Model file for the job. Use its own axes, mm. A direction names the side the tool comes from. Give positions to 0.01 mm unless a question says otherwise; leave off trailing zeros. Order: outer loops, then holes, each group sorted by start corner. A loop starts at its lowest first (then second) coordinate and runs counter-clockwise, first axis right, second up. Notation, with made-up numbers: M 64,22.25 L 116,22.25 A4 ccw 116,29.25 Z; hole C -8.5,48.25 d10. An arc over 180 degrees is marked long. Return JSON: item names as keys, results as strings. Group by question number.
1. Slice it at A-A on z = 4. List the corners of the cut face in (x, y) (3 decimals).
2. Pin check, flat tips, straight feed: pin 1 (14 mm diameter, centred on y = -14, z = 17, fed in from -X); pin 2 (1.5 mm diameter, centred on x = 60, y = 23.5, fed in from -Z); pin 3 (5 mm diameter, centred on y = 15, z = 17.5, fed in from -X) (3 decimals). Stop position of each tip, or through.
3. Slice it at B-B on x = 62.5. List the corners of the cut face in (y, z) (3 decimals), then the cut area to 3 significant figures.
4. Wall check: probe 1 along Y at (x, z) = (24, 44.5); probe 2 along Y at (x, z) = (46, 47.5); probe 3 along Z at (x, y) = (95, 19) (3 decimals). Give the ranges that are in metal, low to high. Write a range as [from, to].
5. 3-axis set-ups, long thin cutter, end or side, ignore diameter. For faces 1 (the face through (59, -24, 42.875)), 2 (the face through (76, 0, 38.1)), 3 (the face through (22.225, 17, 18)), 4 (the face through (54.094, 21.154, 42.578)): which of +Z, -Z, +X, -X, +Y, -Y reach the whole face in a straight line?
6. Two-plate mould, pull along X, no slides. Class faces 5 (the face through (-41.275, -1, 0)), 6 (the face through (41.275, -1, 4)), 7 (the face through (-5, -7.938, 30)), 8 (the face through (59, 24, 42.875)): released by +X, released by -X, zero draft, split by the parting line, or undercut.
from build123d import *

# Parameters (mm, degrees)
F1_DEPTH = 63.5
F2_DEPTH = 25.4
F3_DEPTH = 7.9375
F5_R     = 6.35


with BuildPart() as f1:
    # F0 (on Front) → F1 (new body, symmetric)
    with BuildSketch(Plane.XZ):
        Polygon((22.225, 9.525), (-41.275, 9.525), (-41.275, -9.525), (41.275, -9.525), (41.275, 9.525), align=None)
    extrude(amount=F1_DEPTH, both=True)

    # F0 (on Front) → F2 (join, symmetric)
    with BuildSketch(Plane.XZ):
        with BuildLine():
            Line((22.225, 27.0002), (22.225, 9.525))
            Line((22.225, 9.525), (41.275, 9.525))
            Line((41.275, 9.525), (41.275, 27.0002))
            ThreePointArc((41.275, 27.0002), (44.310306, 36.336039), (52.255521, 42.101846))
            Line((52.255521, 42.101846), (52.255521, 61.416567))
            add(Edge.make_bspline(
                [(50.030877, 61.19192), (50.770384, 61.266108), (51.511964, 61.34093), (52.255521, 61.416567)],
                knots=[106.14327, 106.14327, 106.14327, 106.14327, 107.828168, 107.828168, 107.828168, 107.828168], degree=3))
            ThreePointArc((50.030877, 61.19192), (30.053958, 49.035629), (22.225, 27.0002))
        make_face()
        with BuildLine():
            add(Edge.make_bspline(
                [(52.255521, 61.416567), (53.877929, 61.581604), (55.509751, 61.750523), (57.15, 61.9252)],
                knots=[107.828168, 107.828168, 107.828168, 107.828168, 111.504536, 111.504536, 111.504536, 111.504536], degree=3))
            Line((52.255521, 61.416567), (52.255521, 42.101846))
            ThreePointArc((52.255521, 42.101846), (54.6724, 42.68067), (57.15, 42.8752))
            Line((57.15, 42.8752), (75.536245, 42.8752))
            Line((75.536245, 42.8752), (75.536245, 61.9252))
            Line((75.536245, 61.9252), (57.15, 61.9252))
        make_face()
    extrude(amount=F2_DEPTH, both=True)

    # F0 (on Front) → F3 (join, symmetric)
    with BuildSketch(Plane.XZ):
        with BuildLine():
            add(Edge.make_bspline(
                [(-41.275, 9.525), (-34.917098, 54.362489), (3.444235, 56.518327), (50.030877, 61.19192)],
                knots=[0, 0, 0, 0, 106.14327, 106.14327, 106.14327, 106.14327], degree=3))
            Line((-41.275, 9.525), (22.225, 9.525))
            Line((22.225, 9.525), (22.225, 27.0002))
            ThreePointArc((22.225, 27.0002), (30.053958, 49.035629), (50.030877, 61.19192))
        make_face()
    extrude(amount=F3_DEPTH, both=True)

    # F0 (on Front) → F4 (revolve)
    with BuildSketch(Plane.XZ):
        Polygon((103.055521, 66.675), (75.536245, 66.675), (75.536245, 61.9252), (75.536245, 42.8752), (75.536245, 38.1), (103.055521, 38.1), align=None)
    revolve(axis=Axis((75.536245, 0, 52.3875), (0, 0, 1)))

    # F5
    f5_edges = [f1.edges().sort_by_distance(p)[0] for p in [
        (41.275, -63.5, 0),
        (-41.275, -63.5, 0),
        (41.275, 63.5, 0),
        (-41.275, 63.5, 0),
    ]]
    fillet(f5_edges, radius=F5_R)


solid = f1.part
Result:
{
 "1": {"outline": "M -41.275,-57.15 A6.35 ccw -34.925,-63.5 L 34.925,-63.5 A6.35 ccw 41.275,-57.15 L 41.275,57.15 A6.35 ccw 34.925,63.5 L -34.925,63.5 A6.35 ccw -41.275,57.15 Z"},
 "2": {"pin 1": "stops at x = -40.61", "pin 2": "stops at z = 38.1", "pin 3": "stops at x = 22.225"},
 "3": {"outline": "M -25.4,42.875 L -24.236,42.875 L -24.236,38.1 L 24.236,38.1 L 24.236,42.875 L 25.4,42.875 L 25.4,61.925 L 24.236,61.925 L 24.236,66.675 L -24.236,66.675 L -24.236,61.925 L -25.4,61.925 Z", "area": "1,430 mm2"},
 "4": {"probe 1": "y = [-7.94, 7.94]", "probe 2": "y = [-25.4, 25.4]", "probe 3": "z = [38.1, 66.675]"},
 "5": {"face 1": "-Z, -Y", "face 2": "-Z, +X, +Y, -Y", "face 3": "+Z, -X, +Y", "face 4": "-Z, +Y"},
 "6": {"face 5": "released by -X", "face 6": "released by +X", "face 7": "zero draft", "face 8": "undercut"}
}
